Geometry: final body of the model. Coordinates: model frame, mm. A direction names the side the tool comes from. Round coordinates to 2 decimals unless told otherwise and drop trailing zeros. Write each loop counter-clockwise with the first axis right and the second up, starting at its lowest first coordinate (ties: lowest second). Pieces come first, ordered by that corner, then holes. Notation, with made-up numbers: (-19.5, 88) -> (35.5, 88) arc R18 ccw to (35.5, 121) -> close; hole circle Ø7 at (6, 64). An arc over 180 degrees is marked (long way). One line per item, written item: value. Start each with the question number.
from build123d import *

# Parameters (mm, degrees)
BOSS_EXTRUDE1_DEPTH = 8
SKETCH9_W           = 166
SKETCH9_H           = 57
CUT_EXTRUDE5_DEPTH  = 6
SKETCH10_W          = 10
SKETCH10_H          = 1
CUT_EXTRUDE6_DEPTH  = 6
BOSS_EXTRUDE4_DEPTH = 130
SKETCH13_R          = 3
SKETCH13_W          = 73
SKETCH13_H          = 25
CUT_EXTRUDE7_DEPTH  = 130


with BuildPart() as part:
    # Sketch1 → Boss-Extrude1 (new body)
    with BuildSketch(Plane(origin=(0, 0, 0), x_dir=(1, 0, 0), z_dir=(0, 1, 0))):
        Polygon((0, 0), (88, 0), (170, 0), (170, 41), (170, 61), (0, 61), align=None)
    extrude(amount=BOSS_EXTRUDE1_DEPTH)

    # Sketch9 → Cut-Extrude5 (cut)
    with BuildSketch(Plane.XZ):
        with Locations((85, -30.5)):
            Rectangle(SKETCH9_W, SKETCH9_H)
    extrude(amount=-CUT_EXTRUDE5_DEPTH, mode=Mode.SUBTRACT)

    # Sketch10 → Cut-Extrude6 (cut)
    with BuildSketch(Plane.XZ):
        with Locations((27, -1.5)):
            Rectangle(SKETCH10_W, SKETCH10_H)
        with Locations((27, -59.5)):
            Rectangle(SKETCH10_W, SKETCH10_H)
        with Locations((143, -59.5)):
            Rectangle(SKETCH10_W, SKETCH10_H)
        with Locations((143, -1.5)):
            Rectangle(SKETCH10_W, SKETCH10_H)
    extrude(amount=-CUT_EXTRUDE6_DEPTH, mode=Mode.SUBTRACT)

    # Sketch11 → Boss-Extrude4 (add)
    with BuildSketch(Plane(origin=(22, 0, 0), x_dir=(0, 0, -1), z_dir=(1, 0, 0))):
        Polygon((1, 3.292893219), (1, 4.5), (1.353553391, 4.146446609), (1.353553391, 3.646446609), align=None)
        Polygon((60, 3.292893219), (60, 4.5), (59.646446609, 4.146446609), (59.646446609, 3.646446609), align=None)
    extrude(amount=BOSS_EXTRUDE4_DEPTH)

    # Sketch13 → Cut-Extrude7 (cut)
    with BuildSketch(Plane(origin=(0, 8, 0), x_dir=(1, 0, 0), z_dir=(0, 1, 0))):
        with Locations((18.71505207, 19.7)):
            Circle(SKETCH13_R)
        with Locations((77.5, 19.7)):
            Rectangle(SKETCH13_W, SKETCH13_H)
    extrude(amount=-CUT_EXTRUDE7_DEPTH, mode=Mode.SUBTRACT)


solid = part.part
(1) Line query: probe 1 along X at (y, z) = (6.65, -19.7); probe 2 along X at (y, z) = (2, -24); probe 3 along Z at (x, y) = (56, 7.5). Output: solid intervals per line, ascending.
(2) Section query D-D (z = -51.5). Output: boundary loops of the cut face in (x, y), and give its area (3 significant figures).
(3) Set-up query: faces 4 (the face through (168, 3, -31)), 5 (the face through (84, 8, -38)). Return all of +Z, -Z, +X, -X, +Y, -Y with unobstructed straight access to the full face (end or side cutting, diameter ignored); none if empty.
(4) Pull-direction query (X, two-part tool) for faces 1 (the face through (170, 4, -30)), 2 (the face through (27, 2, -60)), 3 (the face through (85, 0, -60)); classes: pulls with the +X half, pulls with the -X half, needs draft (parallel to the pull), parting line crosses it, or undercut.
(5) Section query A-A (z = -19.7). Output: boundary loops of the cut face in (x, y).
(6) Section query B-B (x = 157.5). Output: boundary loops of the cut face in (y, z), and give its area (3 significant figures).
(7) Section query C-C (z = -10). Output: boundary loops of the cut face in (x, y), and give its area (3 significant figures).
Results list:
1. probe 1: x = 0 to 15.72, 21.72 to 41, 114 to 170
1. probe 2: x = 0 to 2, 168 to 170
1. probe 3: z = -61 to -32.2, -7.2 to 0
2. outline: (0, 0) -> (2, 0) -> (2, 6) -> (168, 6) -> (168, 0) -> (170, 0) -> (170, 8) -> (0, 8) -> close
2. area: 364 mm^2
3. face 4: -Y
3. face 5: +Z, -Z, +X, -X, +Y
4. face 1: pulls with the +X half
4. face 2: undercut
4. face 3: needs draft
5. outline: (0, 0) -> (2, 0) -> (2, 6) -> (15.72, 6) -> (15.72, 8) -> (0, 8) -> close; (21.72, 6) -> (41, 6) -> (41, 8) -> (21.72, 8) -> close; (114, 6) -> (168, 6) -> (168, 0) -> (170, 0) -> (170, 8) -> (114, 8) -> close
6. outline: (0, -61) -> (8, -61) -> (8, 0) -> (0, 0) -> (0, -2) -> (6, -2) -> (6, -59) -> (0, -59) -> close
6. area: 146 mm^2
7. outline: (0, 0) -> (2, 0) -> (2, 6) -> (41, 6) -> (41, 8) -> (0, 8) -> close; (114, 6) -> (168, 6) -> (168, 0) -> (170, 0) -> (170, 8) -> (114, 8) -> close
7. area: 218 mm^2
